Verification items for the finished model (mm, model axes). Face numbers are marked on the shaded views. A direction names the side the tool comes from. Give positions to 0.01 mm unless a question says otherwise; leave off trailing zeros. Order: outer loops, then holes, each group sorted by start corner. A loop starts at its lowest first (then second) coordinate and runs counter-clockwise, first axis right, second up. Notation, with made-up numbers: (-7, 39) -> (32, 39) arc R11 ccw to (32, 46) -> close; hole circle Ø6 at (-35, 30.5). An arc over 180 degrees is marked (long way). Return JSON: item names as keys, results as strings. Group by question number.
(1) Depth check by flat-ended pin: pin 1 Ø5 at (x, y) = (-5, 17) entering from -Z; pin 2 Ø4.5 at (y, z) = (-2, 64) entering from -X; pin 3 Ø2 at (x, y) = (-17, 8.5) entering from -Z. Enter the tip coordinate at first touch or a pass-through.
(2) Cross-section at D-D on x = 0. Enter the section's corners in (y, z), then the cut area to 3 significant figures.
(3) Tool access check on the marked faces 4, 5 and 6. Record the directions out of +Z, -Z, +X, -X, +Y, -Y that give a thin tool (end or side, any length) a straight path to the whole face; none if there is none.
(4) Cross-section at B-B on z = 1.5. Enter the section's corners in (x, y).
(5) Thickness scan on line 1 along Z through (x, y) = (0, 12.25); line 2 along Z through (x, y) = (2, 24); line 3 along X through (y, z) = (19, 62.5). Record the ranges inside material, lowest first.
(6) Release check for a two-part mould opening along Z. For the marked faces 1, 2 and 3 record: pulls with the +Z half, pulls with the -Z half, needs draft (parallel to the pull), parting line crosses it, or undercut.
(7) Cross-section at C-C on z = 28.5. Enter the section's corners in (x, y).
(8) Cross-section at A-A on y = 8. State how many separate pieces and enclosed holes the cut face has, then the cut area to 3 significant figures.
Autodesk Inventor part; units mm, degrees
ref_plane "YZ Plane" through (0, 0, 0) normal (1, 0, 0) x (0, 1, 0)
ref_plane "XY Plane" through (0, 0, 0) normal (0, 0, 1) x (1, 0, 0)
sketch "Sketch1" plane through (0, 0, 0) normal (0, 1, 0) x (-1, 0, 0)
  circle A0 centre (0, 0) radius 10
  circle A1 centre (0, 0) radius 12.5
  line L0 (12.5, 0) -> (12.5, 50)
  line L1 (-12.5, 0) -> (-12.5, 50)
  line L2 (-12.5, 50) -> (12.5, 50)
  dimension "d0" = 20
  dimension "d1" = 25
  dimension "d2" = 50
extrude "Extrusion1" add sketch "Sketch1" along normal blind 15
sketch "Sketch2" plane through (-12.5, 0, 0) normal (-1, 0, 0) x (0, 0, 1)
  line L0 (-12.5, 0) -> (-12.5, 15)
  line L1 (-12.5, 7.5) -> (37.5, 7.5)
  line L2 (25, 7.5) -> (25, 4.5)
  line L3 (25, 4.5) -> (25, 10.5)
  line L4 (25, 10.5) -> (75, 10.5)
  line L5 (75, 10.5) -> (75, 4.5)
  line L6 (75, 4.5) -> (25, 4.5)
  point P0 (0, 0)
  dimension "d5" = 50
  dimension "d8" = 3
  dimension "d9" = 6
  dimension "d10" = 50
extrude "Extrusion2" add sketch "Sketch2" along normal blind 10
sketch "Sketch3" plane through (-12.5, 0, 50) normal (0, 0, 1) x (1, 0, 0)
  point P0 (12.5, 0)
sketch "Sketch4" plane through (-12.5, 0, 50) normal (0, 0, 1) x (1, 0, 0)
  line L0 (25, 0) -> (25, 15)
  line L1 (25, 0) -> (25, 15)
  line L2 (0, 15) -> (25, 15)
  line L3 (25, 15) -> (0, 15)
  line L4 (0, 0) -> (0, 15)
  line L5 (0, 15) -> (0, 0)
  line L6 (0, 0) -> (25, 0)
  line L7 (0, 0) -> (25, 0)
  point P0 (12.5, 0)
extrude "Extrusion3" add sketch "Sketch4" along normal blind 25
sketch "Sketch5" plane through (-12.5, 4.5, 25) normal (0, -1, 0) x (1, 0, 0)
  point P0 (12.5, -25)
sketch "Sketch8" plane through (-12.5, 4.5, 25) normal (0, -1, 0) x (1, 0, 0)
  line L0 (0, 0) -> (-10, 0)
  line L1 (-5, 0) -> (-5, 50)
  line L2 (0, 50) -> (-10, 50)
  line L3 (-3, 12) -> (-7, 12)
  line L4 (-7, 12) -> (-7, 8)
  line L5 (-7, 8) -> (-3, 8)
  line L6 (-3, 8) -> (-3, 12)
  line L7 (-3, 12) -> (-7, 8) construction
  line L8 (-7, 12) -> (-3, 8) construction
  line L9 (-5, 10) -> (-5, 23)
  line L10 (-7, 21) -> (-3, 21)
  line L11 (-3, 21) -> (-3, 25)
  line L12 (-3, 25) -> (-7, 25)
  line L13 (-7, 25) -> (-7, 21)
  line L14 (-7, 21) -> (-3, 25) construction
  line L15 (-3, 21) -> (-7, 25) construction
  line L16 (-5, 23) -> (-5, 36)
  line L17 (-7, 34) -> (-3, 34)
  line L18 (-3, 34) -> (-3, 38)
  line L19 (-3, 38) -> (-7, 38)
  line L20 (-7, 38) -> (-7, 34)
  line L21 (-7, 34) -> (-3, 38) construction
  line L22 (-3, 34) -> (-7, 38) construction
  point P0 (12.5, -25)
  dimension "d40" = 4
  dimension "d41" = 4
  dimension "d42" = 13
  dimension "d43" = 4
  dimension "d44" = 4
  dimension "d45" = 13
  dimension "d46" = 4
  dimension "d47" = 4
extrude "Extrusion6" cut sketch "Sketch8" against normal blind 10
sketch "Sketch9" plane through (0, 0, 0) normal (0, -1, 0) x (1, 0, 0)
  line L0 (-12.5, 25) -> (-22.5, 25)
  line L1 (-12.5, 25) -> (12.5, 25)
  line L2 (12.5, 0) -> (12.5, 75)
  line L3 (-12.5, 25) -> (-12.5, 75)
  line L4 (-12.5, 25) -> (-12.5, 75)
  line L5 (-12.5, 75) -> (12.5, 75)
  line L6 (-12.5, 75) -> (12.5, 75)
  line L7 (12.5, 75) -> (12.5, 25)
  line L8 (12.5, 0) -> (12.5, 30)
  line L9 (-12.5, 25) -> (-10.5, 25)
  line L10 (-10.5, 25) -> (-10.5, 75)
  line L11 (-12.5, 75) -> (-12.5, 25)
  line L12 (-10.5, 25) -> (12.5, 30)
  point P0 (0, 0)
  dimension "d50" = 30
  dimension "d51" = 2
extrude "Extrusion7" add sketch "Sketch9" along normal blind 13 contours L10 L5 L2 L12
sketch "Sketch10" plane through (0, -13, 0) normal (0, -1, 0) x (1, 0, 0)
  point P0 (0, 0)
sketch "Sketch11" plane through (0, -13, 0) normal (0, -1, 0) x (1, 0, 0)
  line L0 (-10.5, 25) -> (12.5, 30)
  line L1 (12.5, 30) -> (-10.5, 30)
  line L2 (-10.5, 25) -> (-10.5, 75)
  line L3 (-10.5, 30) -> (1, 30)
  line L4 (1, 30) -> (1, 75)
  line L5 (12.5, 75) -> (-12.5, 75)
  line L6 (-1, 42) -> (3, 42)
  line L7 (3, 42) -> (3, 38)
  line L8 (3, 38) -> (-1, 38)
  line L9 (-1, 38) -> (-1, 42)
  line L10 (-1, 42) -> (3, 38) construction
  line L11 (3, 42) -> (-1, 38) construction
  line L12 (1, 40) -> (1, 52.5)
  line L13 (-1, 50.5) -> (3, 50.5)
  line L14 (3, 50.5) -> (3, 54.5)
  line L15 (3, 54.5) -> (-1, 54.5)
  line L16 (-1, 54.5) -> (-1, 50.5)
  line L17 (-1, 50.5) -> (3, 54.5) construction
  line L18 (3, 50.5) -> (-1, 54.5) construction
  line L19 (1, 52.5) -> (1, 65)
  line L20 (-1, 63) -> (3, 63)
  line L21 (3, 63) -> (3, 67)
  line L22 (3, 67) -> (-1, 67)
  line L23 (-1, 67) -> (-1, 63)
  line L24 (-1, 63) -> (3, 67) construction
  line L25 (3, 63) -> (-1, 67) construction
  line L26 (-1, 38) -> (-1, 42)
  line L27 (-1, 38) -> (3, 38)
  line L28 (3, 38) -> (3, 42)
  line L29 (3, 42) -> (-1, 42)
  line L30 (-1, 42) -> (-1, 38)
  line L31 (-1, 38) -> (3, 42) construction
  line L32 (3, 38) -> (-1, 42) construction
  point P0 (0, 0)
  dimension "d54" = 11.5
  dimension "d55" = 4
  dimension "d56" = 4
  dimension "d57" = 12.5
  dimension "d58" = 4
  dimension "d59" = 4
  dimension "d60" = 12.5
  dimension "d61" = 4
  dimension "d62" = 4
extrude "Extrusion8" cut sketch "Sketch11" against normal blind 50 contours L8 L9 L6 L4 | L4 L6 L7 L8 | L22 L21 L20 L4 | L4 L20 L23 L22 | L13 L16 L15 L4 | L4 L15 L14 L13
ref_plane "Work Plane1" through (0, 7.5, 0) normal (0, 1, 0) x (-1, 0, 0)
mirror "Mirror1" about plane through (0, 7.5, 0) normal (0, 1, 0) of "Extrusion7"
mirror "Mirror2" about plane through (0, 7.5, 0) normal (0, 1, 0) of "Extrusion8"
properties part number "Part10copy"
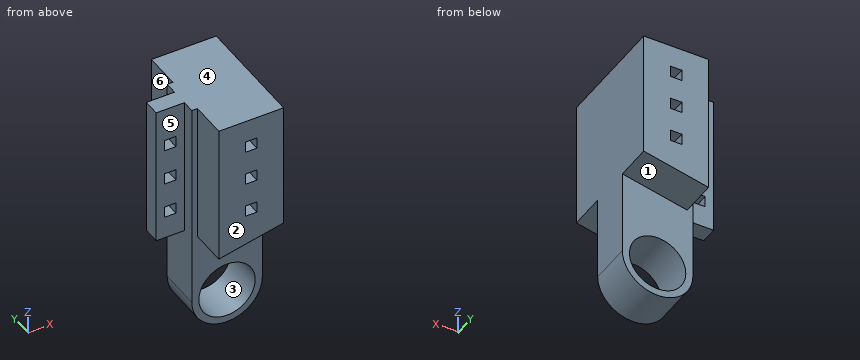
Verdict:
{
 "1": {"pin 1": "z = -12", "pin 2": "x = -12.5", "pin 3": "z = 25"},
 "2": {"outline": "(-13, 27.28) -> (0, 27.28) -> (0, 10) -> (15, 10) -> (15, 27.28) -> (28, 27.28) -> (28, 38) -> (-13, 38) -> close; (-13, 42) -> (28, 42) -> (28, 50.5) -> (-13, 50.5) -> close; (-13, 54.5) -> (28, 54.5) -> (28, 63) -> (-13, 63) -> close; (-13, 67) -> (28, 67) -> (28, 75) -> (-13, 75) -> close; (0, -12.5) -> (15, -12.5) -> (15, -10) -> (0, -10) -> close", "area": "1,760 mm²"},
 "3": {"face 4": "+Z, +X, -X, +Y, -Y", "face 5": "+Z, -Z, -X, -Y", "face 6": "+Z, -Z, -X, +Y"},
 "4": {"outline": "(-12.5, 0) -> (-9.89, 0) -> (-9.89, 15) -> (-12.5, 15) -> close; (9.89, 0) -> (12.5, 0) -> (12.5, 15) -> (9.89, 15) -> close"},
 "5": {"line 1": "-12.5 to -10, 10 to 38, 42 to 50.5, 54.5 to 63, 67 to 75", "line 2": "27.72 to 38, 42 to 50.5, 54.5 to 63, 67 to 75", "line 3": "-10.5 to 12.5"},
 "6": {"face 1": "pulls with the -Z half", "face 2": "needs draft", "face 3": "undercut"},
 "7": {"outline": "(-22.5, 4.5) -> (-12.5, 4.5) -> (-12.5, 0) -> (-10.5, 0) -> (-10.5, -13) -> (5.6, -13) -> (5.6, 0) -> (12.5, 0) -> (12.5, 15) -> (5.6, 15) -> (5.6, 28) -> (-10.5, 28) -> (-10.5, 15) -> (-12.5, 15) -> (-12.5, 10.5) -> (-22.5, 10.5) -> close"},
 "8": {"separate pieces": "1", "enclosed holes": "7", "area": "2,210 mm²"}
}
